from build123d import *

# Parameters (mm, degrees)
SKETCH_W        = 120
SKETCH_H        = 80
PAD_DEPTH       = 1.5
SKETCH001_W     = 117
SKETCH001_H     = 77
PAD001_DEPTH    = 4
POCKET_DEPTH    = 4
SKETCH003_W     = 4
SKETCH003_H     = 4
POCKET001_DEPTH = 1.5
SKETCH004_W     = 4
SKETCH004_H     = 4
POCKET002_DEPTH = 1.5
FILLET_R        = 2
FILLET001_R     = 2
FILLET002_R     = 2
FILLET003_R     = 2
SKETCH005_R     = 1.5
POCKET003_DEPTH = 1.5
SKETCH006_R     = 1.5
POCKET004_DEPTH = 1.5
SKETCH007_R     = 1.5
POCKET005_DEPTH = 1.5
SKETCH008_R     = 1.5
POCKET006_DEPTH = 1.5


with BuildPart() as part:
    # Sketch → Pad (new body)
    with BuildSketch(Plane.XY):
        with Locations((24.76931, 10.449721)):
            Rectangle(SKETCH_W, SKETCH_H)
    extrude(amount=PAD_DEPTH)

    # Sketch001 (on Face6 of Pad) → Pad001 (join)
    with BuildSketch(Plane.XY.offset(1.5)):
        with Locations((24.76931, 10.449721)):
            Rectangle(SKETCH001_W, SKETCH001_H)
    extrude(amount=PAD001_DEPTH)

    # Sketch002 (on Face11 of Pad001) → Pocket (cut)
    with BuildSketch(Plane.XY.offset(5.5)):
        Polygon((81.26931, 46.966207), (81.26931, -26.050279), (64.26931, -26.050279), (64.26931, -24.050279), (58.26931, -24.050279), (58.26931, -26.050279), (-8.73069, -26.050279), (-8.73069, -24.050279), (-14.73069, -24.050279), (-14.73069, -26.050279), (-31.73069, -26.050279), (-31.73069, 46.949721), (-14.73069, 46.949721), (-14.73069, 44.949721), (-8.73069, 44.949721), (-8.73069, 46.949721), (58.26931, 46.949721), (58.26931, 44.966207), (64.26931, 44.966207), (64.26931, 46.966207), align=None)
    extrude(amount=-POCKET_DEPTH, mode=Mode.SUBTRACT)

    # Sketch003 (on Face9 of Pocket) → Pocket001 (cut)
    with BuildSketch(Plane.XZ.offset(28.050279)):
        with Locations((-11.73069, 3.5)):
            Rectangle(SKETCH003_W, SKETCH003_H)
        with Locations((61.26931, 3.5)):
            Rectangle(SKETCH003_W, SKETCH003_H)
    extrude(amount=-POCKET001_DEPTH, mode=Mode.SUBTRACT)

    # Sketch004 (on Face7 of Pocket001) → Pocket002 (cut)
    with BuildSketch(Plane(origin=(0, 48.949721, 0), x_dir=(-1, 0, 0), z_dir=(0, 1, 0))):
        with Locations((-61.26931, 3.5)):
            Rectangle(SKETCH004_W, SKETCH004_H)
        with Locations((11.73069, 3.5)):
            Rectangle(SKETCH004_W, SKETCH004_H)
    extrude(amount=-POCKET002_DEPTH, mode=Mode.SUBTRACT)

    # Fillet
    fillet_edges = [part.edges().sort_by_distance(p)[0] for p in [
        (-33.73069, 48.949721, 3.5),
    ]]
    fillet(fillet_edges, radius=FILLET_R)

    # Fillet001
    fillet001_edges = [part.edges().sort_by_distance(p)[0] for p in [
        (83.26931, 48.949721, 3.5),
    ]]
    fillet(fillet001_edges, radius=FILLET001_R)

    # Fillet002
    fillet002_edges = [part.edges().sort_by_distance(p)[0] for p in [
        (83.26931, -28.050279, 3.5),
    ]]
    fillet(fillet002_edges, radius=FILLET002_R)

    # Fillet003
    fillet003_edges = [part.edges().sort_by_distance(p)[0] for p in [
        (-33.73069, -28.050279, 3.5),
    ]]
    fillet(fillet003_edges, radius=FILLET003_R)

    # Sketch005 (on Face25 of Fillet003) → Pocket003 (cut)
    with BuildSketch(Plane.XZ.offset(26.550279)):
        with Locations((-11.73069, 3.5)):
            Circle(SKETCH005_R)
    extrude(amount=-POCKET003_DEPTH, mode=Mode.SUBTRACT)

    # Sketch006 (on Face28 of Pocket003) → Pocket004 (cut)
    with BuildSketch(Plane.XZ.offset(26.550279)):
        with Locations((61.26931, 3.5)):
            Circle(SKETCH006_R)
    extrude(amount=-POCKET004_DEPTH, mode=Mode.SUBTRACT)

    # Sketch007 (on Face34 of Pocket004) → Pocket005 (cut)
    with BuildSketch(Plane(origin=(0, 47.449721, 0), x_dir=(-1, 0, 0), z_dir=(0, 1, 0))):
        with Locations((-61.26931, 3.5)):
            Circle(SKETCH007_R)
    extrude(amount=-POCKET005_DEPTH, mode=Mode.SUBTRACT)

    # Sketch008 (on Face31 of Pocket005) → Pocket006 (cut)
    with BuildSketch(Plane(origin=(0, 47.449721, 0), x_dir=(-1, 0, 0), z_dir=(0, 1, 0))):
        with Locations((11.73069, 3.5)):
            Circle(SKETCH008_R)
    extrude(amount=-POCKET006_DEPTH, mode=Mode.SUBTRACT)


solid = part.part
Geometry check sheet. Reference: the model listing, model coordinates, mm. A direction names the side the tool comes from. Round coordinates to 2 decimals unless told otherwise and drop trailing zeros. Order: outer loops, then holes, each group sorted by start corner. A loop starts at its lowest first (then second) coordinate and runs counter-clockwise, first axis right, second up. Notation, with made-up numbers: (30.5, 70.5) -> (47.5, 70.5) arc R13 ccw to (47.5, 91.5) -> close; hole circle Ø8 at (-4.75, 54.5). An arc over 180 degrees is marked (long way). Use one line per item in the form item = value.
1. Cross-section at B-B, the plane y = 3.5. Enter the section's corners in (x, z).
Working result:
outline = (-35.23, 0) -> (84.77, 0) -> (84.77, 1.5) -> (83.27, 1.5) -> (83.27, 5.5) -> (81.27, 5.5) -> (81.27, 1.5) -> (-31.73, 1.5) -> (-31.73, 5.5) -> (-33.73, 5.5) -> (-33.73, 1.5) -> (-35.23, 1.5) -> close
2. Cross-section at A-A, the plane x = 56.5. Enter the section's corners in (y, z), plus the area to 3 significant figures.
Working result:
outline = (-29.55, 0) -> (50.45, 0) -> (50.45, 1.5) -> (48.95, 1.5) -> (48.95, 5.5) -> (46.95, 5.5) -> (46.95, 1.5) -> (-26.05, 1.5) -> (-26.05, 5.5) -> (-28.05, 5.5) -> (-28.05, 1.5) -> (-29.55, 1.5) -> close
area = 136 mm^2
3. Mould release check, pull along Z, two halves, no side actions. Record for faces 1 (the face through (24, 11, 0)), 2 (the face through (72, 48.95, 3)), 3 (the face through (-10.232, 46.71, 3.566)): pulls with the +Z half, pulls with the -Z half, needs draft (parallel to the pull), parting line crosses it, or undercut.
Working result:
face_1 = pulls with the -Z half
face_2 = needs draft
face_3 = undercut
4. Go/stop test with flat-tipped pins: pin 1 (0.6 mm diameter, centred on y = -25.5, z = 4, fed in from -X); pin 2 (4 mm diameter, centred on x = 9, y = 14, fed in from +Z); pin 3 (2 mm diameter, centred on x = 61.5, z = 4, fed in from -Y). Record where each tip stops, or that it passes through.
Working result:
pin_1 = -33.73
pin_2 = 1.5
pin_3 = -26.55
5. Scan lines: line 1 along Y through (x, z) = (-13, 2.5); line 2 along Y through (x, z) = (56.5, 1.6); line 3 along X through (y, z) = (34, 1.85). Record each from-to range of solid material in increasing order. Write a range as from..to.
Working result:
line_1 = -26.55..-24.05, 44.95..47.45
line_2 = -28.05..-26.05, 46.95..48.95
line_3 = -33.73..-31.73, 81.27..83.27
6. Set-up check for faces 4 (the face through (-10.345, -25.811, 2.925)), 5 (the face through (-23, -28.05, 3)), 6 (the face through (-23, -26.05, 4)): record each of +Z, -Z, +X, -X, +Y, -Y from which the full face is reachable in a straight line by a thin tool's end or side.
Working result:
face_4 = -Y
face_5 = +Z, +X, -X, -Y
face_6 = +Z
